Design review of the part built by this model. Coordinates are the model's own, in mm. Face numbers are marked on the shaded views. A direction names the side the tool comes from. Coordinates: 2 decimals unless noted, no trailing zeros. Write each loop counter-clockwise with the first axis right and the second up, starting at its lowest first coordinate (ties: lowest second). Pieces come first, ordered by that corner, then holes. Notation, with made-up numbers: (78.25, -0.5) -> (94.25, -0.5) arc R15 ccw to (94.25, 17.5) -> close; hole circle Ø2 at (-27, 15.5). An arc over 180 degrees is marked (long way). Write item = value, one per line. Start each with the question number.
```python
from build123d import *

# Parameters (mm, degrees)
CIRPATTERN1_COUNT = 2
CIRPATTERN1_ANGLE = 90
CIRPATTERN2_COUNT = 2
CIRPATTERN2_ANGLE = 90


with BuildPart() as part:
    # Sketch1 → Revolve1 (revolve)
    with BuildSketch(Plane.XY, mode=Mode.PRIVATE) as revolve1_sk:
        Polygon((0, 0), (0, 12.5), (-141.026059686, 12.5), (-141.026059686, 27.5), (-200, 0), align=None)
    revolve1 = revolve(revolve1_sk.sketch.rotate(Axis((0, 0, 0), (1, 0, 0)), 90), axis=Axis((0, 0, 0), (1, 0, 0)))

    # CirPattern1: Revolve1 ×2 about axis
    cirpattern1_axis = Axis((0, 30.25, 0), (0, 1, 0))
    for i in range(1, CIRPATTERN1_COUNT):
        add(revolve1.rotate(cirpattern1_axis, i * CIRPATTERN1_ANGLE / (CIRPATTERN1_COUNT - 1)))

    # CirPattern2: Revolve1 ×2 about axis
    cirpattern2_axis = Axis((0, 0, -36.375), (0, 0, -1))
    for i in range(1, CIRPATTERN2_COUNT):
        add(revolve1.rotate(cirpattern2_axis, i * CIRPATTERN2_ANGLE / (CIRPATTERN2_COUNT - 1)))

    # Sketch2 → Revolve2 (revolve)
    with BuildSketch(Plane.XY):
        with BuildLine():
            Line((-29.583426204, 0), (29.583426204, 0))
            ThreePointArc((29.583426204, 0), (0, -29.583426204), (-29.583426204, 0))
        make_face()
    revolve(axis=Axis((-29.583426204, 0, 0), (1, 0, 0)))


solid = part.part
```
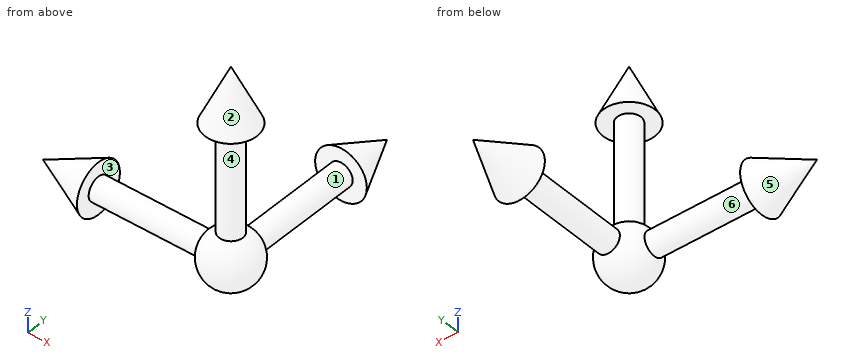
(1) For the marked faces 5 and 6, list the 3-axis set-ups (+Z, -Z, +X, -X, +Y, -Y) from which the entire face can be reached by the end or side of a thin tool; tool diameter is ignored.
(2) Mouldability with a two-part tool opening along Z and no side actions: class the marked faces 1, 2, 3 and 4 as pulls with the +Z half, pulls with the -Z half, needs draft (parallel to the pull), parting line crosses it, or undercut.
(3) For pin 1 Ø10 at (x, y) = (4, 73.5) entering from -Z; pin 2 Ø5 at (x, z) = (-82, 11) entering from -Y; pin 3 Ø10 at (x, y) = (-158.5, -5) entering from +Z, all flat-tipped, find the tip position at first contact; note any pin that passes through.
(4) For line 1 (X direction, y = -14, z = -14.5); line 2 (Z direction, x = 8, y = 20); line 3 (Y direction, x = 12, z = -9), list the stretches that pass through material, from the lowest coordinate up.
(5) Take a section at A-A, the plane z = 48. State the section outline as (x, y) points, then the cut area to 3 significant figures.
Report:
q1.face_5 = -X
q1.face_6 = none
q2.face_1 = parting line crosses it
q2.face_2 = pulls with the +Z half
q2.face_3 = needs draft
q2.face_4 = undercut
q3.pin_1 = -12.5
q3.pin_2 = -9.17
q3.pin_3 = 21.29
q4.line_1 = -156.78 to -141.03, -21.65 to 21.65
q4.line_2 = -20.28 to 20.28, 141.03 to 153.81
q4.line_3 = -25.5 to 25.5, 141.03 to 167.83
q5.outline = circle Ø25 at (0, 0)
q5.area = 491 mm2
